For this review, take the finished solid that the model builds, in its own axes (mm). Face numbers are marked on the shaded views. Coordinates: 2 decimals unless noted, no trailing zeros. Write each loop counter-clockwise with the first axis right and the second up, starting at its lowest first coordinate (ties: lowest second). Pieces come first, ordered by that corner, then holes.
1) We need section C-C on x = 40. Write out the cut boundary in (y, z), then the cut area to 3 significant figures.
2) We need section D-D on y = 7. Write out the cut boundary in (x, z), then the cut area to 3 significant figures.
3) To check wall thickness, follow line 1 along X through (y, z) = (1.05, 0) (3 decimals); line 2 along X through (y, z) = (6.1, 0). State the ranges of each line that lie inside material, in increasing order.
4) We need section A-A on x = 0. Write out the cut boundary in (y, z).
5) Insertion check: P1, Ø4, axis at x = 30.05, z = -30.05, coming from the -Y side; P2, Ø4, axis at x = -23, y = 7.5, coming from the -Z side; P3, Ø1, axis at y = 3.5, z = -29, coming from the +X side; P4, Ø12, axis at x = -38, z = -0.5, coming from the +Y side. Each pin has a flat end and moves straight along its axis. Give the tip position at first contact, or say it passes through.
6) We need section B-B on z = -42.5. Write out the cut boundary in (x, y) (3 decimals), then the cut area to 3 significant figures.
7) Mouldability with a two-part tool opening along Z and no side actions: class the marked faces 1 and 2 as pulls with the +Z half, pulls with the -Z half, needs draft (parallel to the pull), parting line crosses it, or undercut.
from build123d import *

# Parameters (mm, degrees)
SKETCH_1_R                  = 51
SKETCH_1_R_2                = 19
EXTRUDE_1_DEPTH             = 4
PATTERN_CIRCULAR_1_COUNT    = 6
HOLE_WIZARD_M32_D           = 3.15
PATTERN_LINEAR_1_COUNT      = 2
PATTERN_LINEAR_1_PITCH      = 18
PATTERN_LINEAR_1_COUNT_DIR2 = 2
PATTERN_LINEAR_1_PITCH_DIR2 = 85
SKETCH_14_R                 = 28
SKETCH_14_R_2               = 26
EXTRUDE_2_DEPTH             = 5
SKETCH_16_R                 = 1.5
SKETCH_16_W                 = 9
SKETCH_16_H                 = 26
CUT_EXTRUDE_1_DEPTH         = 5
FILLET_1_R                  = 2
PATTERN_CIRCULAR_2_COUNT    = 4


with BuildPart() as part:
    # Эскиз1 → Бобышка-Вытянуть1 (new body)
    with BuildSketch(Plane(origin=(0, 0, 0), x_dir=(1, 0, 0), z_dir=(0, 1, 0))):
        Circle(SKETCH_1_R)
        Circle(SKETCH_1_R_2, mode=Mode.SUBTRACT)
    extrude(amount=EXTRUDE_1_DEPTH)

    # Эскиз3 → Сверло под метчик  спиральное M2.51 (revolve, cut)
    with BuildSketch(Plane(origin=(23.5, 4, 0), x_dir=(0, 0, 1), z_dir=(1, 0, 0))):
        Polygon((0, 0), (0, 8.766097289), (1.275, 8), (1.275, 0), align=None)
    hole_wizard_m2_51 = revolve(axis=Axis((23.5, 10.35, 0), (0, -1, 0)), mode=Mode.SUBTRACT)

    # Круговой массив1: Сверло под метчик  спиральное M2.51 ×6 about axis
    pattern_circular_1_axis = Axis((0, 0, 0), (0, 1, 0))
    for i in range(1, PATTERN_CIRCULAR_1_COUNT):
        add(hole_wizard_m2_51.rotate(pattern_circular_1_axis, i * 360 / PATTERN_CIRCULAR_1_COUNT), mode=Mode.SUBTRACT)

    # Сверло под метчик  спиральное M32 (through all)
    with Locations(Plane(origin=(0, 0, 0), x_dir=(-1, 0, 0), z_dir=(0, -1, 0))):
        with Locations((-9, -42.5)):
            hole_wizard_m32 = Hole(HOLE_WIZARD_M32_D / 2)

    # Линейный массив1: Hole Wizard M32 2 × 2
    with Locations(*[(-i * PATTERN_LINEAR_1_PITCH, 0, -j * PATTERN_LINEAR_1_PITCH_DIR2) for i in range(PATTERN_LINEAR_1_COUNT) for j in range(PATTERN_LINEAR_1_COUNT_DIR2) if (i, j) != (0, 0)]):
        add(hole_wizard_m32, mode=Mode.SUBTRACT)

    # Эскиз14 → Бобышка-Вытянуть2 (add)
    with BuildSketch(Plane(origin=(0, 4, 0), x_dir=(1, 0, 0), z_dir=(0, 1, 0))):
        Circle(SKETCH_14_R)
        Circle(SKETCH_14_R_2, mode=Mode.SUBTRACT)
    extrude(amount=EXTRUDE_2_DEPTH)

    # Эскиз16 → Вырез-Вытянуть1 (cut, through all)
    with BuildSketch(Plane(origin=(0, 4, 0), x_dir=(1, 0, 0), z_dir=(0, 1, 0))):
        with Locations((40, 16.82)):
            Circle(SKETCH_16_R)
        with Locations((40, -16.82)):
            Circle(SKETCH_16_R)
        with Locations((40, 0)):
            Rectangle(SKETCH_16_W, SKETCH_16_H)
    extrude(amount=-CUT_EXTRUDE_1_DEPTH, mode=Mode.SUBTRACT)

    # Скругление1
    fillet_1_edges = [part.edges().sort_by_distance(p)[0] for p in [
        (35.5, 2, 13),
        (35.5, 2, -13),
        (44.5, 2, -13),
        (44.5, 2, 13),
    ]]
    fillet(fillet_1_edges, radius=FILLET_1_R)

    # Эскиз18 → Сверло под метчик  спиральное M51 (revolve, cut)
    with BuildSketch(Plane(origin=(-30.0520382, 4, -30.0520382), x_dir=(0, 0, 1), z_dir=(1, 0, 0))):
        Polygon((0, 0), (0, 9.562237609), (2.6, 8), (2.6, 0), align=None)
    hole_wizard_m51 = revolve(axis=Axis((-30.0520382, 10.35, -30.0520382), (0, -1, 0)), mode=Mode.SUBTRACT)

    # Круговой массив2: Сверло под метчик  спиральное M51 ×4 about axis
    pattern_circular_2_axis = Axis((0, 0, 0), (0, 1, 0))
    for i in range(1, PATTERN_CIRCULAR_2_COUNT):
        add(hole_wizard_m51.rotate(pattern_circular_2_axis, i * 360 / PATTERN_CIRCULAR_2_COUNT), mode=Mode.SUBTRACT)


solid = part.part
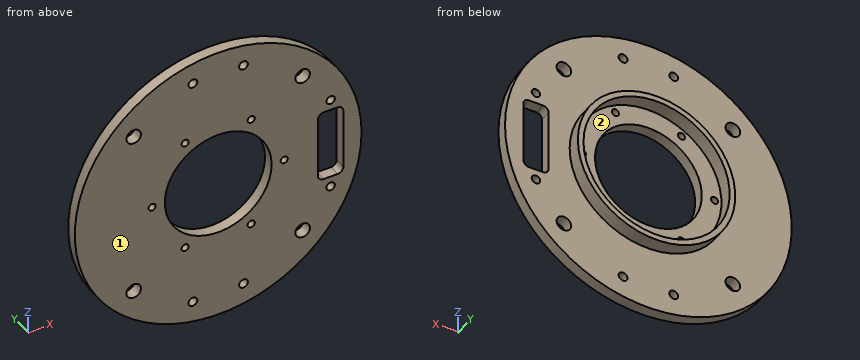
Result:
1. outline: (0, -31.64) - (4, -31.64) - (4, -18.32) - (0, -18.32) - close; (0, -15.32) - (4, -15.32) - (4, -13) - (0, -13) - close; (0, 13) - (4, 13) - (4, 15.32) - (0, 15.32) - close; (0, 18.32) - (4, 18.32) - (4, 31.64) - (0, 31.64) - close
1. area: 125 mm2
2. outline: circle Ø56 at (0, 0); hole circle Ø52 at (0, 0)
2. area: 339 mm2
3. line 1: x = -51 to -24.775, -22.225 to -19, 19 to 22.225, 24.775 to 35.5, 44.5 to 51
3. line 2: x = -28 to -26, 26 to 28
4. outline: (0, -51) - (4, -51) - (4, -28) - (9, -28) - (9, -26) - (4, -26) - (4, -19) - (0, -19) - close; (0, 19) - (4, 19) - (4, 26) - (9, 26) - (9, 28) - (4, 28) - (4, 51) - (0, 51) - close
5. P1: passes through
5. P2: stops at z = -18.52
5. P3: stops at x = 42.29
5. P4: stops at y = 4
6. outline: (-28.191, 0) - (-10.575, 0) - (-10.575, 4) - (-28.191, 4) - close; (-7.425, 0) - (7.425, 0) - (7.425, 4) - (-7.425, 4) - close; (10.575, 0) - (28.191, 0) - (28.191, 4) - (10.575, 4) - close
6. area: 200 mm2
7. face 1: needs draft
7. face 2: undercut
